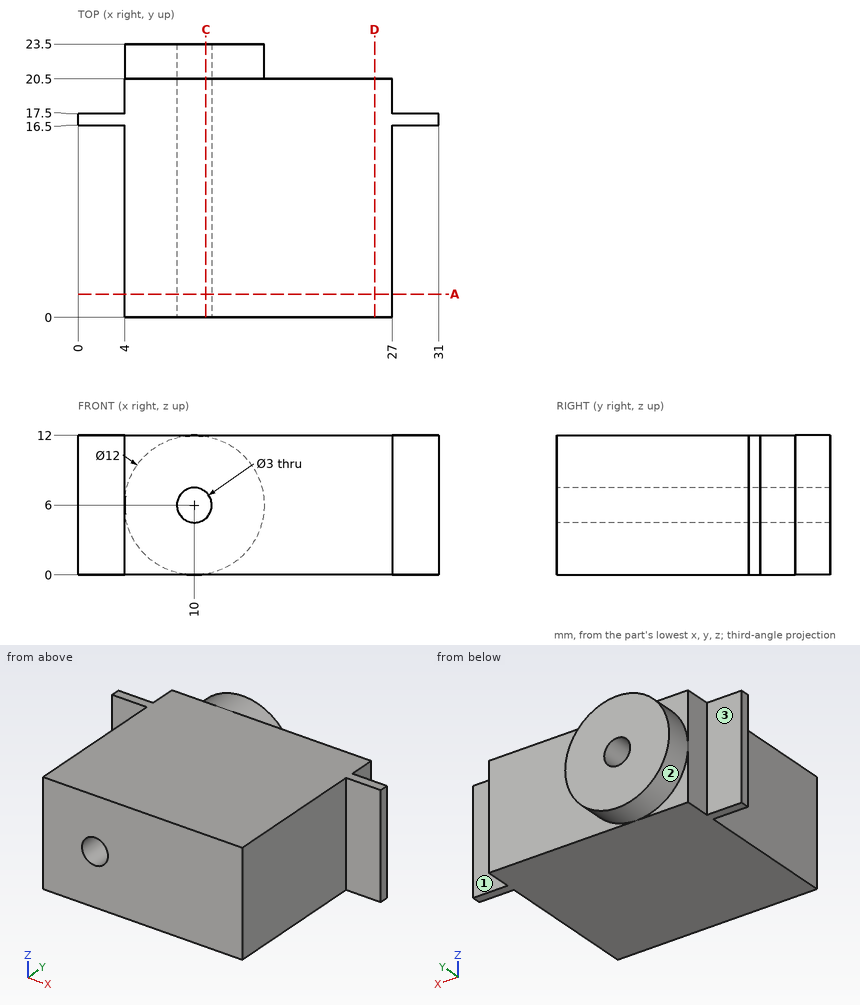
Input: dimensioned drawing with shaded views. Units: mm. Origin: part minimum x, y, z. A direction names the side the tool comes from. Coordinates: 2 decimals unless noted, no trailing zeros. Write each loop counter-clockwise with the first axis right and the second up, starting at its lowest first coordinate (ties: lowest second). Pieces come first, ordered by that corner, then holes. Notation, with made-up numbers: M 80.25,-0.5 L 93.25,-0.5 A19 cw 93.25,11.5 Z; hole C 52,-37 d10. An arc over 180 degrees is marked long. Answer as a JSON object with one key per item and string values. Group by question number.
(1) Contact query for flat-ended pins moving along their axis: P1, Ø1.2, axis at x = 3, z = 6.5, coming from the -Y side; P2, Ø4, axis at x = 17.5, z = 10, coming from the +Y side; P3, Ø1.2, axis at x = 2, z = 6, coming from the +Y side; P4, Ø2.5, axis at x = 10, z = 6, coming from the -Y side. Output: stop coordinate, or through.
(2) Section D-D on x = 25.5. Output: boundary loops of the cut face in (y, z).
(3) Section C-C on x = 11. Output: boundary loops of the cut face in (y, z), plus the area to 3 significant figures.
(4) Ray query, line 1 along X through (y, z) = (16.75, 6); line 2 along X through (y, z) = (9.5, 6); line 3 along Z through (x, y) = (10, 6.5). Return the intervals inside material, ascending. Write a range as [from, to].
(5) Set-up query: the marked faces 1, 2 and 3. Return all of +Z, -Z, +X, -X, +Y, -Y with unobstructed straight access to the full face (end or side cutting, diameter ignored); none if empty.
(6) Section A-A on y = 2. Output: boundary loops of the cut face in (x, z).
Result set:
{
 "1": {"P1": "stops at y = 16.5", "P2": "stops at y = 20.5", "P3": "stops at y = 17.5", "P4": "passes through"},
 "2": {"outline": "M 0,0 L 20.5,0 L 20.5,12 L 0,12 Z"},
 "3": {"outline": "M 0,0 L 20.5,0 L 20.5,0.08 L 23.5,0.08 L 23.5,4.88 L 0,4.88 Z; M 0,7.12 L 23.5,7.12 L 23.5,11.92 L 20.5,11.92 L 20.5,12 L 0,12 Z", "area": "229 mm2"},
 "4": {"line 1": "x = [0, 8.5], [11.5, 31]", "line 2": "x = [4, 8.5], [11.5, 27]", "line 3": "z = [0, 4.5], [7.5, 12]"},
 "5": {"face 1": "+Z, -Z, +X, +Y", "face 2": "+Y", "face 3": "+Z, -Z, -X, +Y"},
 "6": {"outline": "M 4,0 L 27,0 L 27,12 L 4,12 Z; hole C 10,6 d3"}
}
